The model under review builds one solid part; all positions refer to its coordinate system, in mm. Face numbers are marked on the shaded views. A direction names the side the tool comes from. Give positions to 0.01 mm unless a question says otherwise; leave off trailing zeros. Loops run counter-clockwise (first coordinate to the right, second up) from the corner with the lowest first, then second, coordinate; pieces in that order, holes last. Notation, with made-up numbers: (20, 73) - (73, 73) arc R32 ccw to (73, 103) - close; hole circle Ø5 at (52, 25.25). An arc over 180 degrees is marked (long way). Return JSON: item names as keys, results as strings. Group by question number.
from build123d import *

# Parameters (mm, degrees)
F0_R     = 10.795
F1_DEPTH = 38.1
F3_D     = 3.25
F4_R     = 3
F5_DEPTH = 15.272
F7_DEPTH = 15.272
F8_SIZE  = 1.905
F9_R     = 5.08
F10_R    = 2.54


with BuildPart() as f1:
    # F0 (on Top) → F1 (new body)
    with BuildSketch(Plane.XY):
        with BuildLine():
            ThreePointArc((8.255, 13.2439750453), (3.3583146073, 10.3871947138), (0, 5.8198711326))
            ThreePointArc((0, 5.8198711326), (-3.3583146073, 10.3871947138), (-8.255, 13.2439750453))
            Line((-8.255, 13.2439750453), (-8.255, 17.272))
            Line((-8.255, 17.272), (-17.145, 17.272))
            Line((-17.145, 17.272), (-17.145, 13.2439750453))
            ThreePointArc((-17.145, 13.2439750453), (-26.67, 0), (-17.145, -13.2439750453))
            Line((-17.145, -13.2439750453), (-17.145, -17.272))
            Line((-17.145, -17.272), (-8.255, -17.272))
            Line((-8.255, -17.272), (-8.255, -13.2439750453))
            ThreePointArc((-8.255, -13.2439750453), (-3.3583146073, -10.3871947138), (0, -5.8198711326))
            ThreePointArc((0, -5.8198711326), (3.3583146073, -10.3871947138), (8.255, -13.2439750453))
            Line((8.255, -13.2439750453), (8.255, -17.272))
            Line((8.255, -17.272), (17.145, -17.272))
            Line((17.145, -17.272), (17.145, -13.2439750453))
            ThreePointArc((17.145, -13.2439750453), (26.67, 0), (17.145, 13.2439750453))
            Line((17.145, 13.2439750453), (17.145, 17.272))
            Line((17.145, 17.272), (8.255, 17.272))
            Line((8.255, 17.272), (8.255, 13.2439750453))
        make_face()
        with Locations((-12.7, 0)):
            Circle(F0_R, mode=Mode.SUBTRACT)
        with Locations((12.7, 0)):
            Circle(F0_R, mode=Mode.SUBTRACT)
    extrude(amount=F1_DEPTH)

    # F3 (through all)
    with Locations(Plane.XZ.offset(17.272)):
        with Locations((-12.7, 31.75), (12.7, 31.75), (12.7, 6.35), (-12.7, 6.35)):
            Hole(F3_D / 2)

    # F4 (on Front) → F5 (cut, through all)
    with BuildSketch(Plane.XZ):
        with Locations((-12.7, 31.75)):
            Circle(F4_R)
        with Locations((-12.7, 6.35)):
            Circle(F4_R)
        with Locations((12.7, 6.35)):
            Circle(F4_R)
        with Locations((12.7, 31.75)):
            Circle(F4_R)
    extrude(amount=-F5_DEPTH, mode=Mode.SUBTRACT)

    # F6 (on Front) → F7 (cut, through all)
    with BuildSketch(Plane.XZ):
        Polygon((-9.9568, 30.1662127416), (-9.9568, 33.3337872584), (-12.7, 34.9175745169), (-15.4432, 33.3337872584), (-15.4432, 30.1662127416), (-12.7, 28.5824254831), align=None)
        Polygon((-9.9568, 4.7662127416), (-9.9568, 7.9337872584), (-12.7, 9.5175745169), (-15.4432, 7.9337872584), (-15.4432, 4.7662127416), (-12.7, 3.1824254831), align=None)
        Polygon((15.4432, 4.7662127416), (15.4432, 7.9337872584), (12.7, 9.5175745169), (9.9568, 7.9337872584), (9.9568, 4.7662127416), (12.7, 3.1824254831), align=None)
        Polygon((15.4432, 30.1662127416), (15.4432, 33.3337872584), (12.7, 34.9175745169), (9.9568, 33.3337872584), (9.9568, 30.1662127416), (12.7, 28.5824254831), align=None)
    extrude(amount=F7_DEPTH, mode=Mode.SUBTRACT)

    # F8
    f8_edges = [f1.edges().sort_by_distance(p)[0] for p in [
        (12.7, -17.272, 38.1),
        (12.7, -17.272, 0),
        (-12.7, -17.272, 0),
        (-12.7, -17.272, 38.1),
        (12.7, 17.272, 38.1),
        (12.7, 17.272, 0),
        (-12.7, 17.272, 0),
        (-12.7, 17.272, 38.1),
    ]]
    chamfer(f8_edges, length=F8_SIZE)

    # F9
    f9_edges = [f1.edges().sort_by_distance(p)[0] for p in [
        (0, 5.819871, 19.05),
        (0, -5.819871, 19.05),
    ]]
    fillet(f9_edges, radius=F9_R)

    # F10
    f10_edges = [f1.edges().sort_by_distance(p)[0] for p in [
        (-8.255, -13.243975, 19.05),
        (8.255, -13.243975, 19.05),
        (17.145, -13.243975, 19.05),
        (17.145, 13.243975, 19.05),
        (8.255, 13.243975, 19.05),
        (-17.145, 13.243975, 19.05),
        (-8.255, 13.243975, 19.05),
        (-17.145, -13.243975, 19.05),
    ]]
    fillet(f10_edges, radius=F10_R)


solid = f1.part
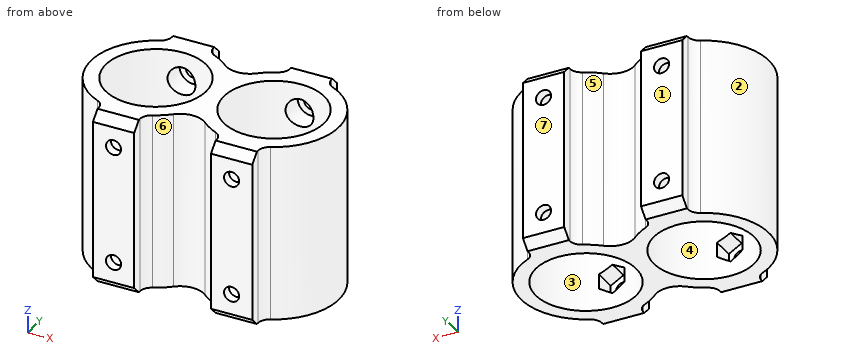
Item 1: Mouldability with a two-part tool opening along Y and no side actions: class the marked faces 1, 2, 3 and 4 as +Y half, -Y half, draft (parallel to the pull), parting line (faces both ways), or undercut.
Item 2: Take a section at B-B (y = -12). State how many separate pieces and enclosed holes the cut face has, then the cut area to 3 significant figures.
Item 3: For L1, parallel to X at y = 12.2, z = 31.75; L2, parallel to X at y = -7, z = 11; L3, parallel to X at y = -4, z = 12.5, list the stretches that pass through material, from the lowest coordinate up. Write a range as from..to.
Item 4: Tool access review of the marked faces 5, 6 and 7: name each direction out of +Z, -Z, +X, -X, +Y, -Y from which nothing blocks a thin tool from reaching the whole face with its end or side.
Item 5: For P1, Ø4, axis at y = -10.5, z = 13.5, coming from the +X side; P2, Ø2.5, axis at x = -12.7, z = 31.75, coming from the -Y side; P3, Ø8, axis at x = -4, z = 12, coming from the -Y side; P4, Ø1.6, axis at y = -12.5, z = 6, coming from the -X side, all flat-tipped, find the tip position at first contact; note any pin that passes through.
Item 6: Take a section at C-C (x = -9). State the section outline as (y, z) points (3 decimals).
Item 7: Take a section at A-A (y = 0). State the section outline as (x, z) points (3 decimals), then the cut area to 3 significant figures.
Check sheet entries:
{
 "1": {"face 1": "+Y half", "face 2": "parting line", "face 3": "undercut", "face 4": "undercut"},
 "2": {"separate pieces": "2", "enclosed holes": "4", "area": "986 mm^2"},
 "3": {"L1": "x = -19.51..-15.7, -9.7..-5.89, 5.89..9.7, 15.7..19.51", "L2": "x = -24.79..-20.92, -4.48..4.48, 20.92..24.79", "L3": "x = -26.09..-22.73, -2.67..2.67, 22.73..26.09"},
 "4": {"face 5": "+Z, -Z, +Y", "face 6": "+Z, -Z, -Y", "face 7": "+Z, -Z, +X, -X, +Y"},
 "5": {"P1": "stops at x = 23.79", "P2": "passes through", "P3": "stops at y = -13.85", "P4": "stops at x = -20.33"},
 "6": {"outline": "(-17.272, 1.905) - (-15.367, 0) - (-10.141, 0) - (-10.141, 38.1) - (-15.367, 38.1) - (-17.272, 36.195) - close; (10.141, 0) - (15.367, 0) - (17.272, 1.905) - (17.272, 36.195) - (15.367, 38.1) - (10.141, 38.1) - close"},
 "7": {"outline": "(-26.67, 0) - (-23.495, 0) - (-23.495, 38.1) - (-26.67, 38.1) - close; (-1.905, 0) - (1.905, 0) - (1.905, 38.1) - (-1.905, 38.1) - close; (23.495, 0) - (26.67, 0) - (26.67, 38.1) - (23.495, 38.1) - close", "area": "387 mm^2"}
}
